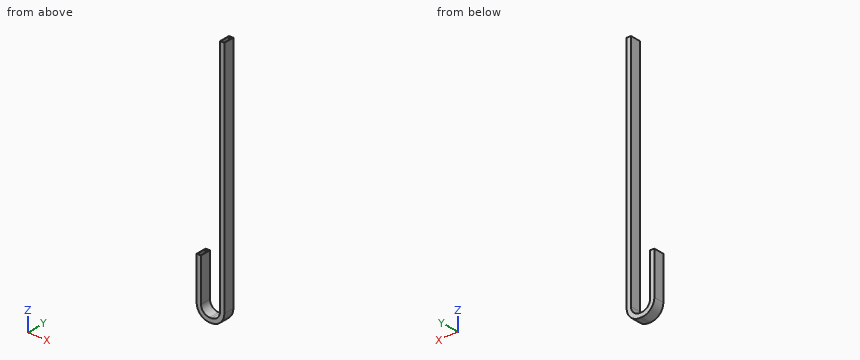
from build123d import *

# Parameters (mm, degrees)
SKETCH1_W      = 14.986
SKETCH1_H      = 37.084
SKETCH1_W_2    = 11.811
SKETCH1_H_2    = 33.909
EXTRUDE1_DEPTH = 12.7
SKETCH2_W      = 14.986
SKETCH2_H      = 37.084
SKETCH2_W_2    = 11.811
SKETCH2_H_2    = 33.909
EXTRUDE2_DEPTH = 12.7
SKETCH3_W      = 14.986
SKETCH3_H      = 37.084
SKETCH3_W_2    = 11.811
SKETCH3_H_2    = 33.909


with BuildPart() as part:
    # Sketch1 → Extrude1 (new body)
    with BuildSketch(Plane.XY):
        with Locations((13.843, 88.392)):
            Rectangle(SKETCH1_W, SKETCH1_H)
        with Locations((13.843, 88.392)):
            Rectangle(SKETCH1_W_2, SKETCH1_H_2, mode=Mode.SUBTRACT)
    extrude(amount=-EXTRUDE1_DEPTH)



with BuildPart() as body_2:
    # Sketch2 → Extrude2 (new body)
    with BuildSketch(Plane.XY.offset(666.75)):
        with Locations((94.107, 88.392)):
            Rectangle(SKETCH2_W, SKETCH2_H)
        with Locations((94.107, 88.392)):
            Rectangle(SKETCH2_W_2, SKETCH2_H_2, mode=Mode.SUBTRACT)
    extrude(amount=-EXTRUDE2_DEPTH)


with BuildPart() as part_1:
    add(part.part)

    add(body_2.part)  # Sweep1 merges body 2
    # Sweep1: sweep along a curve in space
    with BuildLine() as sweep1_path:
        Line((101.6, 69.85, 654.05), (101.6, 69.85, -146.513751223))
        ThreePointArc((101.6, 69.85, -146.513751223), (88.580896424, 69.85, -177.944647647), (57.15, 69.85, -190.963751223))
        Line((57.15, 69.85, -190.963751223), (50.8, 69.85, -190.963751223))
        ThreePointArc((6.35, 69.85, -146.513751223), (19.369103576, 69.85, -177.944647647), (50.8, 69.85, -190.963751223))
        Line((6.35, 69.85, -146.513751223), (6.35, 69.85, -12.7))
    # Sketch3 → Sweep1 (sweep)
    with BuildSketch(Plane(origin=(0, 0, 654.05), x_dir=(-1, 0, 0), z_dir=(0, 0, -1))):
        with Locations((-94.107, 88.392)):
            Rectangle(SKETCH3_W, SKETCH3_H)
        with Locations((-94.107, 88.392)):
            Rectangle(SKETCH3_W_2, SKETCH3_H_2, mode=Mode.SUBTRACT)
    sweep(path=sweep1_path.line)


solid = part_1.part
Geometry: final body of the model. Coordinates: model frame, mm. Give positions to 0.01 mm unless a question says otherwise; leave off trailing zeros. Write each loop counter-clockwise with the first axis right and the second up, starting at its lowest first coordinate (ties: lowest second). Pieces come first, ordered by that corner, then holes. Notation, with made-up numbers: (-19.75, -17) -> (-14.75, -17) arc R24 ccw to (-14.75, -4) -> close; hole circle Ø1 at (50.25, -15.75). An arc over 180 degrees is marked (long way). Answer as a JSON object with one key per item and string values.
1. Cut plane C-C on z = 62. Output: boundary loops of the cut face in (x, y).
Ans:
{"outline": "(86.61, 69.85) -> (101.6, 69.85) -> (101.6, 106.93) -> (86.61, 106.93) -> close; hole (88.2, 71.44) -> (100.01, 71.44) -> (100.01, 105.35) -> (88.2, 105.35) -> close"}
2. Cut plane A-A on z = -92.5. Output: boundary loops of the cut face in (x, y), and give its area (3 significant figures).
Ans:
{"outline": "(6.35, 69.85) -> (21.34, 69.85) -> (21.34, 106.93) -> (6.35, 106.93) -> close; (86.61, 69.85) -> (101.6, 69.85) -> (101.6, 106.93) -> (86.61, 106.93) -> close; hole (7.94, 71.44) -> (19.75, 71.44) -> (19.75, 105.35) -> (7.94, 105.35) -> close; hole (88.2, 71.44) -> (100.01, 71.44) -> (100.01, 105.35) -> (88.2, 105.35) -> close", "area": "310 mm^2"}
3. Cut plane D-D on x = 70.5. Output: boundary loops of the cut face in (y, z), and give its area (3 significant figures).
Ans:
{"outline": "(69.85, -188.91) -> (106.93, -188.91) -> (106.93, -172.78) -> (69.85, -172.78) -> close; hole (71.44, -187.24) -> (105.35, -187.24) -> (105.35, -174.55) -> (71.44, -174.55) -> close", "area": "168 mm^2"}
4. Ray query, probe 1 along Z at (x, y) = (57.5, 87); probe 2 along X at (y, z) = (73.5, -135.5); probe 3 along X at (y, z) = (87.5, 405.5). Return the intervals inside material, ascending. Write a range as from..to.
Ans:
{"probe 1": "z = -190.96..-189.37, -177.56..-175.98", "probe 2": "x = 6.35..7.94, 19.75..21.34, 86.61..88.2, 100.01..101.6", "probe 3": "x = 86.61..88.2, 100.01..101.6"}
5. Contact query for flat-ended pins moving along their axis: pin 1 (12 mm diameter, centred on x = 15.5, y = 95, fed in from +Z); pin 2 (1.9 mm diameter, centred on x = 55.5, y = 82, fed in from +Z); pin 3 (10 mm diameter, centred on y = 83, z = 26.5, fed in from -X). Output: stop coordinate, or through.
Ans:
{"pin 1": "stops at z = 0", "pin 2": "stops at z = -175.98", "pin 3": "stops at x = 86.61"}
